from build123d import *

# Parameters (mm, degrees)
AUFSATZ_LINEAR_AUSTRAGEN1_DEPTH = 3
SCHNITT_LINEAR_AUSTRAGEN1_DEPTH = 1
SCHNITT_LINEAR_AUSTRAGEN2_DEPTH = 1


with BuildPart() as part:
    # Skizze1 → Aufsatz-Linear austragen1 (new body)
    with BuildSketch(Plane.XY):
        with BuildLine():
            Line((2.25, 0), (15.25, 0))
            ThreePointArc((15.25, 0), (16.840990258, 0.659009742), (17.5, 2.25))
            Line((17.5, 2.25), (17.5, 9.25))
            ThreePointArc((17.5, 9.25), (18.159009742, 10.840990258), (19.75, 11.5))
            Line((19.75, 11.5), (20.5, 11.5))
            Line((20.5, 11.5), (20.5, 16))
            Line((20.5, 16), (17.5, 16))
            ThreePointArc((17.5, 16), (15.025126266, 14.974873734), (14, 12.5))
            Line((14, 12.5), (14, 12.25))
            ThreePointArc((14, 12.25), (13.340990258, 10.659009742), (11.75, 10))
            Line((11.75, 10), (2.25, 10))
            ThreePointArc((2.25, 10), (0.659009742, 9.340990258), (0, 7.75))
            Line((0, 7.75), (0, 2.25))
            ThreePointArc((0, 2.25), (0.659009742, 0.659009742), (2.25, 0))
        make_face()
        with BuildLine():
            Line((3.75, 6.75), (13.75, 6.75))
            ThreePointArc((13.75, 6.75), (15.5, 5), (13.75, 3.25))
            Line((13.75, 3.25), (3.75, 3.25))
            ThreePointArc((3.75, 3.25), (2, 5), (3.75, 6.75))
        make_face(mode=Mode.SUBTRACT)
    extrude(amount=AUFSATZ_LINEAR_AUSTRAGEN1_DEPTH)

    # Skizze2 → Schnitt-Linear austragen1 (cut)
    with BuildSketch(Plane(origin=(0, 0, 0), x_dir=(-1, 0, 0), z_dir=(0, 0, -1))):
        Polygon((0.473585846, 10), (-20.5, 10), (-20.5, 11.5), (-20.5, 17.5), (0.473585846, 17.5), (0.473585846, 12.5), align=None)
    extrude(amount=-SCHNITT_LINEAR_AUSTRAGEN1_DEPTH, mode=Mode.SUBTRACT)

    # Skizze3 → Schnitt-Linear austragen2 (cut)
    with BuildSketch(Plane(origin=(0, 0, 0), x_dir=(-1, 0, 0), z_dir=(0, 0, -1))):
        with BuildLine():
            Line((-17.5, 7.8), (-18.826048275, 7.8))
            Line((-18.826048275, 7.8), (-18.826048275, 10.648235291))
            Line((-18.826048275, 10.648235291), (-15.3, 10.648235291))
            Line((-15.3, 10.648235291), (-15.3, 10))
            ThreePointArc((-15.3, 10), (-16.855634919, 9.355634919), (-17.5, 7.8))
        make_face()
    extrude(amount=-SCHNITT_LINEAR_AUSTRAGEN2_DEPTH, mode=Mode.SUBTRACT)


solid = part.part
Source: CAD feature listing. Evaluate the final solid. Frame: model axes, mm. A direction names the side the tool comes from. Give positions to 0.01 mm unless a question says otherwise; leave off trailing zeros. Write each loop counter-clockwise with the first axis right and the second up, starting at its lowest first coordinate (ties: lowest second). Pieces come first, ordered by that corner, then holes. Notation, with made-up numbers: M 15,5.25 L 72,5.25 A20 cw 72,10.25 Z; hole C 74,-40 d3. An arc over 180 degrees is marked long. Return JSON: item names as keys, results as strings. Group by question number.
1) Set-up query: faces 4 (the face through (0.64, 0.68, 1.48)), 5 (the face through (2, 5, 1)), 6 (the face through (17.5, 6, 1)). Return all of +Z, -Z, +X, -X, +Y, -Y with unobstructed straight access to the full face (end or side cutting, diameter ignored); none if empty.
2) Draft query along X for faces 1 (the face through (9, 6.75, 1)), 2 (the face through (13.36, 10.68, 1.99)), 3 (the face through (16.84, 9.37, 0.49)). Return one class per face: released by +X, released by -X, zero draft, split by the parting line, or undercut.
3) First-contact query: pin 1 Ø0.9 at (x, z) = (6.5, 1) entering from +Y; pin 2 Ø2.5 at (x, y) = (14.5, 12) entering from -Z. Flat tips, straight axial feed; report the tip coordinate or a pass-through.
4) Cut plane C-C, the plane z = 2.3. Output: boundary loops of the cut face in (x, y).
5) Ray query, L1, parallel to Y at x = 9.75, z = 0.95; L2, parallel to X at y = 2.5, z = 2.2; L3, parallel to Z at x = 14.5, y = 12.5. Return the intervals inside material, ascending.
6) Cut plane B-B, the plane x = 11.5. Output: boundary loops of the cut face in (y, z).
7) Cut plane D-D, the plane y = 1.5. Output: boundary loops of the cut face in (x, z).
8) Cut plane A-A, the plane y = 5. Output: boundary loops of the cut face in (x, z).
Data:
{
 "1": {"face 4": "+Z, -Z, -X, -Y", "face 5": "+Z, -Z", "face 6": "+Z, -Z, +X, -Y"},
 "2": {"face 1": "undercut", "face 2": "released by -X", "face 3": "released by +X"},
 "3": {"pin 1": "stops at y = 10", "pin 2": "stops at z = 1"},
 "4": {"outline": "M 0,2.25 A2.25 ccw 2.25,0 L 15.25,0 A2.25 ccw 17.5,2.25 L 17.5,9.25 A2.25 cw 19.75,11.5 L 20.5,11.5 L 20.5,16 L 17.5,16 A3.5 ccw 14,12.5 L 14,12.25 A2.25 cw 11.75,10 L 2.25,10 A2.25 ccw 0,7.75 Z; hole M 3.75,3.25 L 13.75,3.25 A1.75 ccw 13.75,6.75 L 3.75,6.75 A1.75 ccw Z"},
 "5": {"L1": "y = 0 to 3.25, 6.75 to 10", "L2": "x = 0 to 17.5", "L3": "z = 1 to 3"},
 "6": {"outline": "M 0,0 L 3.25,0 L 3.25,3 L 0,3 Z; M 6.75,0 L 10,0 L 10,3 L 6.75,3 Z"},
 "7": {"outline": "M 0.13,0 L 17.37,0 L 17.37,3 L 0.13,3 Z"},
 "8": {"outline": "M 0,0 L 2,0 L 2,3 L 0,3 Z; M 15.5,0 L 17.5,0 L 17.5,3 L 15.5,3 Z"}
}
